CAD build for the part. Positions are in the model's coordinates, mm. A direction names the side the tool comes from. Give positions to 0.01 mm unless a question says otherwise; leave off trailing zeros. Loops run counter-clockwise (first coordinate to the right, second up) from the corner with the lowest first, then second, coordinate; pieces in that order, holes last. Notation, with made-up numbers: (29, 19) -> (52, 19) arc R25 ccw to (52, 52) -> close; hole circle Ø3 at (-2.75, 82). An arc over 180 degrees is marked (long way). Use one line per item in the form item = value.
```python
from build123d import *

# Parameters (mm, degrees)
BOSS_EXTRUDE1_DEPTH = 10
SKETCH2_R           = 2.5
BOSS_EXTRUDE2_DEPTH = 8


with BuildPart() as part:
    # Sketch1 → Boss-Extrude1 (new body)
    with BuildSketch(Plane(origin=(0, 0, 0), x_dir=(1, 0, 0), z_dir=(0, 1, 0))):
        Polygon((-5, -17.5), (5, -17.5), (5, 2.5), (15, 2.5), (15, 17.5), (5, 17.5), (-5, 17.5), align=None)
    extrude(amount=BOSS_EXTRUDE1_DEPTH)

    # Sketch2 → Boss-Extrude2 (add)
    with BuildSketch(Plane(origin=(0, 0, -17.5), x_dir=(-1, 0, 0), z_dir=(0, 0, -1))):
        with Locations((-10, 5)):
            Circle(SKETCH2_R)
    extrude(amount=BOSS_EXTRUDE2_DEPTH)


solid = part.part
```
1. Cut at B-B, the plane x = 10. Write the cut outline in (y, z).
Result sheet:
outline = (0, -17.5) -> (2.5, -17.5) -> (2.5, -25.5) -> (7.5, -25.5) -> (7.5, -17.5) -> (10, -17.5) -> (10, -2.5) -> (0, -2.5) -> close
2. Drill centre lines: line 1 (X direction, y = 7.75, z = 7.5); line 2 (Z direction, x = -2, y = 5.5); line 3 (Z direction, x = 11.5, y = 2.5). Where is each one in solid material? Low to high.
Result sheet:
line_1 = -5 to 5
line_2 = -17.5 to 17.5
line_3 = -17.5 to -2.5
3. Cut at A-A, the plane y = 3. Write the cut outline in (x, z), then the cut area to 3 significant figures.
Result sheet:
outline = (-5, -17.5) -> (8.5, -17.5) -> (8.5, -25.5) -> (11.5, -25.5) -> (11.5, -17.5) -> (15, -17.5) -> (15, -2.5) -> (5, -2.5) -> (5, 17.5) -> (-5, 17.5) -> close
area = 524 mm^2
4. Cut at C-C, the plane z = 5.5. Write the cut outline in (x, y), then the cut area to 3 significant figures.
Result sheet:
outline = (-5, 0) -> (5, 0) -> (5, 10) -> (-5, 10) -> close
area = 100 mm^2
5. Cut at D-D, the plane y = 5. Write the cut outline in (x, z), then the cut area to 3 significant figures.
Result sheet:
outline = (-5, -17.5) -> (7.5, -17.5) -> (7.5, -25.5) -> (12.5, -25.5) -> (12.5, -17.5) -> (15, -17.5) -> (15, -2.5) -> (5, -2.5) -> (5, 17.5) -> (-5, 17.5) -> close
area = 540 mm^2
6. Tool access for faces 1 (the flat face through (3, 0, -4)), 2 (the cylindrical face through (11.84, 6.69, -21.44)), 3 (the flat face through (10, 5, -2.5)): list every direction of +Z, -Z, +X, -X, +Y, -Y with a clear straight run to the whole face (end or side of a thin tool).
Result sheet:
face_1 = +Z, -Z, +X, -X, -Y
face_2 = -Z
face_3 = +Z, +X, +Y, -Y
7. Drop flat-ended pins along their axis: P1, Ø5, axis at x = 12, z = -15.5, coming from the -Y side; P2, Ø4, axis at x = 6, z = -21, coming from the +Y side; P3, Ø5, axis at x = 8.5, y = 5.5, coming from the +Z side. Give the stop position or say it passes through.
Result sheet:
P1 = 0
P2 = 6.5
P3 = -2.5
